Verification items for the finished model (mm, model axes). Give positions to 0.01 mm unless a question says otherwise; leave off trailing zeros. Loops run counter-clockwise (first coordinate to the right, second up) from the corner with the lowest first, then second, coordinate; pieces in that order, holes last. Notation, with made-up numbers: (64, 63) -> (118, 63) arc R18 cw to (118, 73) -> close; hole circle Ø8 at (-12, -34). An arc over 180 degrees is marked (long way). Use one line per item in the form item = value. Start each with the question number.
Autodesk Inventor part; units mm, degrees
ref_plane "YZ Plane" through (0, 0, 0) normal (1, 0, 0) x (0, 1, 0)
ref_plane "XZ Plane" through (0, 0, 0) normal (0, 1, 0) x (-1, 0, 0)
ref_plane "XY Plane" through (0, 0, 0) normal (0, 0, 1) x (1, 0, 0)
sketch "スケッチ1" plane through (0, 0, 0) normal (0, 0, 1) x (1, 0, 0)
  line L0 (0, 0) -> (-7.8332, 74.5283) construction
  line L1 (0, 0) -> (0, 134.5604) construction
  circle A0 centre (-16.8762, 26.6318) radius 1 construction
  circle A1 centre (10.9704, 29.5586) radius 1 construction
  line L2 (3.0524, 29.3154) -> (3.3227, 26.7438)
  arc A2 (3.0524, 29.3154) -> (1.4981, 30.5741) centre (2.2753, 29.9448) ccw
  arc A3 (-7.8221, 29.5945) -> (-9.0807, 28.0402) centre (-8.4514, 28.8173) ccw
  line L3 (-8.8105, 25.4686) -> (-9.0807, 28.0402)
  line L4 (13.9144, 27.8571) -> (7.5904, 88.0256) construction
  line L5 (13.9144, 27.8571) -> (28.9995, 61.7387)
  line L6 (-8.8105, 25.4686) -> (-9.2555, 24.9191)
  line L7 (-9.2555, 24.9191) -> (-18.8526, 23.9104)
  line L8 (3.3227, 26.7438) -> (3.8722, 26.2988)
  line L9 (3.8722, 26.2988) -> (13.4694, 27.3075)
  line L10 (-7.8221, 29.5945) -> (1.4981, 30.5741)
  line L11 (3.8722, 26.2988) -> (-9.2555, 24.9191) construction
  arc A4 (-10.8792, -1.6259) -> (-18.8786, 22.5819) centre (-85.0554, -12.7116) ccw construction
  line L12 (13.9144, 27.8571) -> (13.4694, 27.3075)
  line L13 (-19.4021, 24.3553) -> (-18.8526, 23.9104)
  circle A5 centre (3.8901, 77.2154) radius 7.16 construction
  circle A6 centre (-25, 122.4745) radius 9.55 construction
  circle A7 centre (-21.2321, 104.0155) radius 2 construction
  line L14 (-15.9609, 44.2312) -> (-19.3155, 76.1481) construction
  arc A8 (-14.8655, 81.6434) -> (-19.3155, 76.1481) centre (-14.3428, 76.6708) ccw
  line L15 (-14.8655, 81.6434) -> (-2.434, 82.95) construction
  line L16 (3.0613, 78.5) -> (5.9572, 50.9476) construction
  line L17 (4.5173, 71.2482) -> (2.8365, 71.0716)
  line L18 (-2.077, 76.5882) -> (-2.6377, 81.9231)
  arc A9 (-2.077, 76.5882) -> (4.5173, 71.2482) centre (3.8901, 77.2154) ccw
  line L19 (-14.8655, 81.6434) -> (-3.7368, 82.8131)
  line L20 (3.9356, 70.1816) -> (4.9303, 60.7174)
  arc A10 (-2.6377, 81.9231) -> (-3.7368, 82.8131) centre (-3.6323, 81.8185) ccw
  arc A11 (3.9356, 70.1816) -> (2.8365, 71.0716) centre (2.9411, 70.077) ccw
  line L21 (-19.3155, 76.1481) -> (-17.3476, 57.4248)
  circle A12 centre (-3.7775, 43.594) radius 12 construction
  circle A13 centre (-3.7775, 43.594) radius 12.2
  arc A14 (2.2029, 58.6497) -> (-14.0859, 56.0911) centre (-3.7775, 43.594) ccw
  arc A15 (2.2029, 58.6497) -> (4.9303, 60.7174) centre (2.9413, 60.5084) ccw
  arc A16 (-17.3476, 57.4248) -> (-14.0859, 56.0911) centre (-15.3585, 57.6339) ccw
  circle A17 centre (-22.3632, 83.6205) radius 1.3 construction
  circle A18 centre (4.4889, 86.4428) radius 1.3 construction
  circle A19 centre (9.9243, 34.7276) radius 1.3 construction
  circle A20 centre (-16.9277, 31.9053) radius 1.3 construction
  circle A21 centre (-15.447, 110.9099) radius 2.05
  arc A22 (-21.785, 101.8583) -> (-19.4333, 105.2168) centre (-20.6092, 103.5375) ccw
  arc A23 (-19.6004, 105.3375) -> (-19.4333, 105.2168) centre (-15.447, 110.9099) ccw construction
  arc A24 (-20.3614, 105.9955) -> (-23.2605, 103.0964) centre (-21.8109, 104.5459) ccw
  arc A25 (-23.2605, 103.0964) -> (-21.785, 101.8583) centre (-15.447, 110.9099) ccw
  arc A26 (-20.3614, 105.9955) -> (-19.4333, 105.2168) centre (-15.447, 110.9099) ccw
  arc A27 (-15.447, 91.9599) -> (-12.1564, 92.2478) centre (-15.447, 110.9099) ccw
  arc A28 (-11.7917, 90.1797) -> (-12.1564, 92.2478) centre (-11.974, 91.2137) ccw
  arc A29 (-15.447, 89.8599) -> (-11.7917, 90.1797) centre (-15.447, 110.9099) ccw
  arc A30 (-15.447, 91.9599) -> (-15.447, 89.8599) centre (-15.447, 90.9099) ccw
  line L22 (-25, 122.4745) -> (0, 0) construction
  line L23 (28.9995, 61.7387) -> (-17.9684, 153.3176)
  line L24 (-17.9684, 153.3176) -> (-45.126, 132.0122)
  line L25 (-45.126, 132.0122) -> (-19.4021, 24.3553)
  point P0 (3.8311, 71.1761)
  point P1 (-2.7423, 82.9176)
  point P2 (5.3213, 56.9974)
  point P3 (-16.8933, 53.1027)
  point P4 (-16.8933, 53.1027)
  dimension "d0" = 6
  dimension "d1" = 45
  dimension "d2" = 45
  dimension "d3" = 0.5
  dimension "d4" = 45
  dimension "d5" = 45
  dimension "d6" = 6
  dimension "d7" = 1
  dimension "d8" = 0.2
  dimension "d10" = 4
  dimension "d11" = 2
  dimension "d42" = 30
extrude "押し出し1" add sketch "スケッチ1" against normal blind 2
hole "穴1" at (10.9704, 29.5586, 0) at (-16.8762, 26.6318, 0) direction (0, 0, -1) diameter 2 end through all
hole "穴2" at (9.9243, 34.7276, 0) at (4.4889, 86.4428, 0) at (-22.3632, 83.6205, 0) at (-16.9277, 31.9053, 0) direction (0, 0, -1) diameter 2.6 end through all countersink diameter 5.5 countersink angle 90
hole "穴3" at (-25, 122.4745, 0) direction (0, 0, -1) diameter 10 end through all counterbore diameter 11.3 counterbore depth 0.65
hole "穴4" at (3.8901, 77.2154, 0) direction (0, 0, -1) diameter 6 end through all counterbore diameter 7.3 counterbore depth 0.65
properties part number "UPPER_LEG_MIDDLE_FRAME_2"
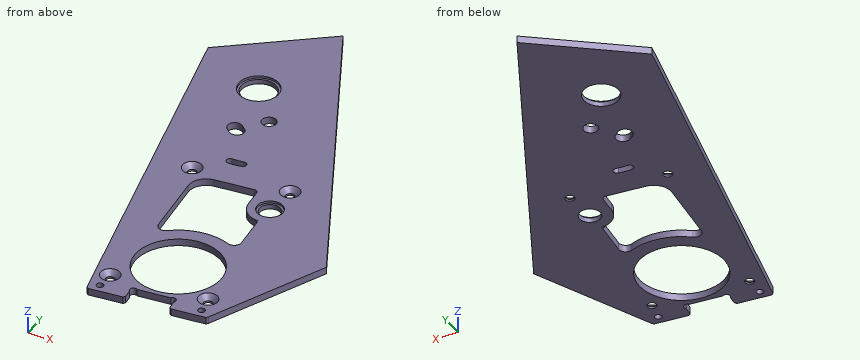
Item 1: Material ranges on line 1 (Y direction, x = -3, z = -0.95); line 2 (Y direction, x = -12, z = -0.35); line 3 (X direction, y = 77, z = -1), recorded low to high.
Item 2: Gauge pin test, flat ends, axial feed: pin 1 Ø3 at (x, y) = (-22.36, 83.62) entering from +Z; pin 2 Ø1 at (x, z) = (-21.5, -1) entering from +Y; pin 3 Ø7 at (x, y) = (3.89, 77.22) entering from +Z; pin 4 Ø1.6 at (x, y) = (9.92, 34.73) entering from -Z. Record the tip position at first contact, or that the pin passes through.
Item 3: Sectioned sample at C-C, the plane x = -39. Enter the section's corners in (y, z), and give its area (3 significant figures).
Item 4: Sectioned sample at A-A, the plane y = 41.5. Enter the section's corners in (x, z).
Item 5: Sectioned sample at B-B, the plane x = 18. Enter the section's corners in (y, z).
Outcome:
q1.line_1 = 30.1 to 31.42, 55.77 to 59.78, 82.59 to 124.13
q1.line_2 = 24.63 to 34.58, 52.61 to 57.55, 81.94 to 90.14, 92.26 to 141.68
q1.line_3 = -31.98 to -19.33, -2.12 to 0.9, 6.88 to 21.17
q2.pin_1 = -1.25
q2.pin_2 = 150.94
q2.pin_3 = -0.65
q2.pin_4 = through
q3.outline = (106.37, -2) -> (136.82, -2) -> (136.82, 0) -> (106.37, 0) -> close
q3.area = 60.9 mm^2
q4.outline = (-23.5, -2) -> (-15.8, -2) -> (-15.8, 0) -> (-23.5, 0) -> close; (8.24, -2) -> (19.99, -2) -> (19.99, 0) -> (8.24, 0) -> close
q5.outline = (37.03, -2) -> (83.19, -2) -> (83.19, 0) -> (37.03, 0) -> close
